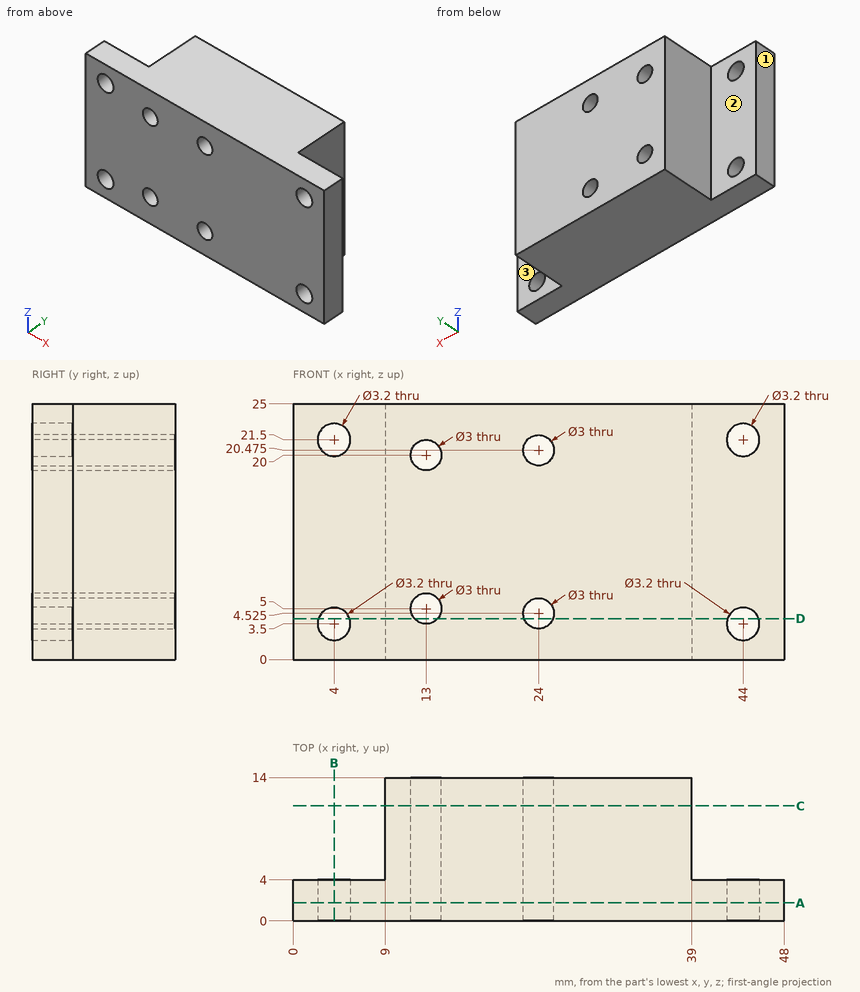
Verification items for this drawing (mm, ordinates from the low corner). A direction names the side the tool comes from. Coordinates: 2 decimals unless noted, no trailing zeros. Loops run counter-clockwise (first coordinate to the right, second up) from the corner with the lowest first, then second, coordinate; pieces in that order, holes last.
Item 1: Sectioned sample at D-D, the plane z = 4. Record the boundary of the cut face in (x, y), then the cut area to 3 significant figures.
Item 2: Sectioned sample at A-A, the plane y = 1.75. Count the separate pieces of the cut face and the enclosed holes in it, then the cut area to 3 significant figures.
Item 3: Go/stop test with flat-tipped pins: pin 1 Ø3 at (y, z) = (9, 9.5) entering from +X; pin 2 Ø2.5 at (x, z) = (4, 3.5) entering from -Y; pin 3 Ø10 at (x, z) = (45.5, 11.5) entering from +Y. Record where each tip stops, or that it passes through.
Item 4: Access from +Z, -Z, +X, -X, +Y, -Y to the whole of each face (thin tool, end or side, straight path). Record for the marked faces 1, 2 and 3.
Item 5: Sectioned sample at C-C, the plane y = 11.25. Record the boundary of the cut face in (x, z) (3 decimals).
Item 6: Thickness scan on line 1 (X direction, y = 5.5, z = 5); line 2 (X direction, y = 4.75, z = 12.5); line 3 (X direction, y = 7, z = 5.25). Record the ranges inside material, lowest first.
Item 7: Sectioned sample at B-B, the plane x = 4. Record the boundary of the cut face in (y, z), then the cut area to 3 significant figures.
Check result:
1. outline: (0, 0) - (2.48, 0) - (2.48, 4) - (0, 4) - close; (5.52, 0) - (11.88, 0) - (11.88, 14) - (9, 14) - (9, 4) - (5.52, 4) - close; (14.12, 0) - (22.59, 0) - (22.59, 14) - (14.12, 14) - close; (25.41, 0) - (42.48, 0) - (42.48, 4) - (39, 4) - (39, 14) - (25.41, 14) - close; (45.52, 0) - (48, 0) - (48, 4) - (45.52, 4) - close
1. area: 397 mm2
2. separate pieces: 1
2. enclosed holes: 8
2. area: 1,140 mm2
3. pin 1: stops at x = 39
3. pin 2: passes through
3. pin 3: stops at y = 4
4. face 1: +Z, -Z, -X, +Y, -Y
4. face 2: +Z, -Z, -X, +Y
4. face 3: +Z, -Z, +X, +Y
5. outline: (9, 0) - (39, 0) - (39, 25) - (9, 25) - close; hole circle Ø3 at (13, 5); hole circle Ø3 at (13, 20); hole circle Ø3 at (24, 4.525); hole circle Ø3 at (24, 20.475)
6. line 1: x = 9 to 11.5, 14.5 to 22.58, 25.42 to 39
6. line 2: x = 9 to 39
6. line 3: x = 9 to 11.52, 14.48 to 22.69, 25.31 to 39
7. outline: (0, 0) - (4, 0) - (4, 1.9) - (0, 1.9) - close; (0, 5.1) - (4, 5.1) - (4, 19.9) - (0, 19.9) - close; (0, 23.1) - (4, 23.1) - (4, 25) - (0, 25) - close
7. area: 74.4 mm2
